The model under review builds one solid part; all positions refer to its coordinate system, in mm. A direction names the side the tool comes from. Coordinates: 2 decimals unless noted, no trailing zeros. Order: outer loops, then holes, each group sorted by start corner. A loop starts at its lowest first (then second) coordinate and runs counter-clockwise, first axis right, second up. Notation, with made-up numbers: (24.5, 77.5) -> (51.5, 77.5) arc R19 cw to (51.5, 112.5) -> close; hole circle Ø8 at (15, -11). An arc over 180 degrees is marked (long way). Use CSV: the item, a comma, the result in double quotes. Start each with the question number.
```python
from build123d import *

# Parameters (mm, degrees)
F2_T            = -1.5
F3_R            = 19.5
F3_R_2          = 11
F4_DEPTH        = 4
F5_R            = 13
F6_DEPTH        = 1
F7_SIZE         = 0.25
F9_D            = 3.2
F9_COPIES_COUNT = 4


# Not quite as in the source:
# - a pattern or mirror of a feature is missing from the dataset's text; its kind, count and spacing are read off the source's solid


with BuildPart() as f1:
    # F0 (on Front) → F1 (revolve)
    with BuildSketch(Plane.XZ):
        with BuildLine():
            Line((-39.0004168703, 0), (0, 0))
            Line((0, 0), (0, 11))
            Line((0, 11), (-13.379, 11))
            ThreePointArc((-13.379, 11), (-24.9848227606, 9.544537302), (-35.8718437294, 5.2682926829))
            ThreePointArc((-35.8718437294, 5.2682926829), (-38.1593199105, 3.0636121528), (-39.0004168703, 0))
        make_face()
    revolve(axis=Axis((-19.5002084352, 0, 0), (1, 0, 0)))

    # F2
    f2_openings = [f1.faces().sort_by_distance(p)[0] for p in [
        (0, 0, 0),
    ]]
    offset(amount=F2_T, openings=f2_openings)

    # F3 (on Right) → F4 (join)
    with BuildSketch(Plane.YZ):
        Circle(F3_R)
        Circle(F3_R_2, mode=Mode.SUBTRACT)
    extrude(amount=-F4_DEPTH)

    # F5 (on Right) → F6 (cut)
    with BuildSketch(Plane.YZ):
        Circle(F5_R)
    extrude(amount=-F6_DEPTH, mode=Mode.SUBTRACT)

    # F7
    f7_edges = [f1.edges().sort_by_distance(p)[0] for p in [
        (-4, -19.5, 0),
        (-4, 0, -11),
        (0, -19.5, 0),
        (0, -13, 0),
    ]]
    chamfer(f7_edges, length=F7_SIZE)

    # F9 (through all)
    with Locations(Plane.YZ):
        with Locations((0, 15)):
            f9 = Hole(F9_D / 2)

    # F9_copies: F9 ×4 about axis
    f9_copies_axis = Axis((0, 0, 0), (1, 0, 0))
    for i in range(1, F9_COPIES_COUNT):
        add(f9.rotate(f9_copies_axis, i * 360 / F9_COPIES_COUNT), mode=Mode.SUBTRACT)


solid = f1.part
```
Q1. For faces 1 (the cylindrical face through (-2.028, -0.208, -16.586)), 2 (the flat face through (-4, 8.3, -8.3)), 3 (the cylindrical face through (-0.62, -10.316, -7.91)), list the 3-axis set-ups (+Z, -Z, +X, -X, +Y, -Y) from which the entire face can be reached by the end or side of a thin tool; tool diameter is ignored.
Q2. Clearance check with flat-ended pins moving along their axes: pin 1 Ø2 at (x, z) = (-6, -2.5) entering from +Y; pin 2 Ø8 at (x, z) = (-19, 0) entering from +Y; pin 3 Ø6 at (x, z) = (-22.5, 14.5) entering from +Y; pin 4 Ø4 at (y, z) = (0, 15) entering from -X. State where each tip first meets the part, or that it passes through.
Q3. Add section A-A, the plane x = -12. State the section outline as (y, z) points.
Q4. To check wall thickness, follow probe 1 along Z at (x, y) = (-0.65, 0); probe 2 along Z at (x, y) = (-2.25, 0); probe 3 along Y at (x, z) = (-5, 0). State the ranges of each line that lie inside material, in increasing order.
Q5. Draft analysis for pull direction Z (two halves, no side actions). For faces 4 (the cylindrical face through (-1.976, -2.539, 19.334)), 5 (the flat face through (0, -5, -13)), 6 (the cylindrical face through (-7.28, 8.43, 4.38)), state which applies: +Z half, -Z half, draft (parallel to the pull), parting line (faces both ways), or undercut.
Answer block:
1,face 1,"+X, -X"
1,face 2,"-X"
1,face 3,"+X"
2,pin 1,"stops at y = 10.9"
2,pin 2,"stops at y = 10.97"
2,pin 3,"passes through"
2,pin 4,"stops at x = -4"
3,outline,"circle Ø22 at (0, 0); hole circle Ø19 at (0, 0)"
4,probe 1,"z = -19.5 to -16.6, -13.4 to -13, 13 to 13.4, 16.6 to 19.5"
4,probe 2,"z = -19.5 to -16.6, -13.4 to -9.5, 9.5 to 13.4, 16.6 to 19.5"
4,probe 3,"y = -11 to -9.5, 9.5 to 11"
5,face 4,"parting line"
5,face 5,"draft"
5,face 6,"undercut"
